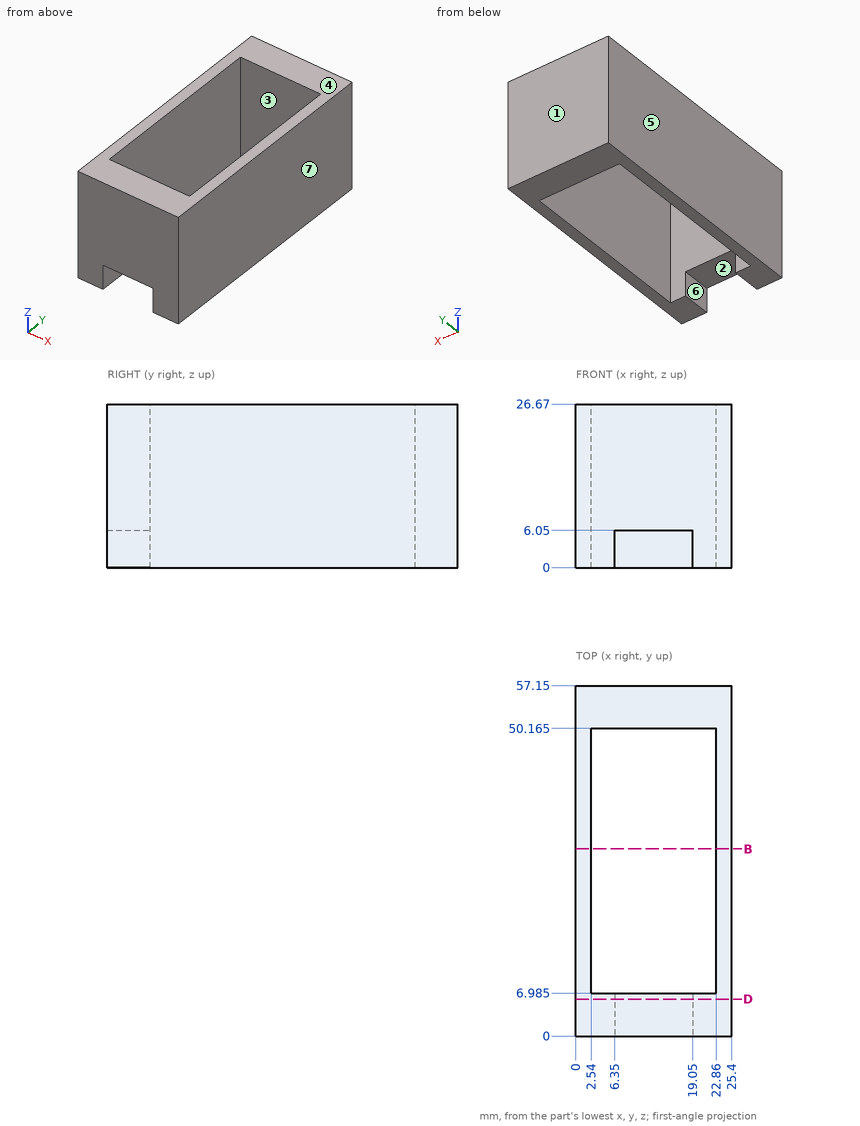
Study the drawing (mm; zero at the part's minimum x, y, z) and answer. A direction names the side the tool comes from. Give positions to 0.01 mm unless a question says otherwise; leave off trailing zeros. Loops run counter-clockwise (first coordinate to the right, second up) from the corner with the lowest first, then second, coordinate; pieces in that order, holes last. Notation, with made-up numbers: M 27,-38.5 L 71,-38.5 A24 cw 71,-2.5 Z; hole C -38,73 d7. An arc over 180 degrees is marked long. One line per item, written item: value. Start each with the question number.
1. Find the intervals of material crossed by probe 1 along X at (y, z) = (10.5, 2.5), in increasing order.
2. Each of these flat-tipped pins is pushed along its axis until it touches: P1, Ø1, axis at x = 7.5, z = 12.5, coming from the -Y side; P2, Ø5, axis at x = 11, z = 3, coming from the -Y side (3 decimals); P3, Ø5.5, axis at x = 11.5, y = 3.5, coming from the -Z side; P4, Ø3, axis at x = 5, y = 45.5, coming from the +Z side. Where does it stop, or does it pass through?
3. Determine the mould class of the marked faces 4, 5, 6 and 7 for opening direction X: released by +X, released by -X, zero draft, split by the parting line, or undercut.
4. Find section B-B (y = 30.5). Give the vertices of the cut face in (x, z).
5. Which of the six approach directions +Z, -Z, +X, -X, +Y, -Y give full straight-line access (tool end or side, diameter ignored) to the marked faces 1, 2 and 3?
6. Find section D-D (y = 6). Give the vertices of the cut face in (x, z).
Reported:
1. probe 1: x = 0 to 2.54, 22.86 to 25.4
2. P1: stops at y = 0
2. P2: stops at y = 50.165
2. P3: stops at z = 6.05
2. P4: passes through
3. face 4: zero draft
3. face 5: released by -X
3. face 6: undercut
3. face 7: released by +X
4. outline: M 0,0 L 2.54,0 L 2.54,26.67 L 0,26.67 Z; M 22.86,0 L 25.4,0 L 25.4,26.67 L 22.86,26.67 Z
5. face 1: +Z, -Z, +X, -X, +Y
5. face 2: -Z, -Y
5. face 3: +Z, -Z
6. outline: M 0,0 L 6.35,0 L 6.35,6.05 L 19.05,6.05 L 19.05,0 L 25.4,0 L 25.4,26.67 L 0,26.67 Z
